```python
from build123d import *

# Parameters (mm, degrees)
SKETCH_1_R      = 2.5
EXTRUDE_1_DEPTH = 2
FILLET_1_R      = 4.5


with BuildPart() as part:
    # 草图1 → 凸台-拉伸1 (new body)
    with BuildSketch(Plane.XY):
        Polygon((-7.5, 7.5), (-7.5, -7.5), (-3, -7.5), (-3, -137.5), (-7.5, -137.5), (-7.5, -152.5), (7.5, -152.5), (7.5, -137.5), (3, -137.5), (3, -7.5), (7.5, -7.5), (7.5, 7.5), align=None)
        Circle(SKETCH_1_R, mode=Mode.SUBTRACT)
        with Locations((0, -145)):
            Circle(SKETCH_1_R, mode=Mode.SUBTRACT)
    extrude(amount=EXTRUDE_1_DEPTH)

    # 圆角1
    fillet_1_edges = [part.edges().sort_by_distance(p)[0] for p in [
        (-7.5, 7.5, 1),
        (-7.5, -7.5, 1),
        (7.5, -7.5, 1),
        (7.5, 7.5, 1),
        (7.5, -152.5, 1),
        (7.5, -137.5, 1),
        (-7.5, -152.5, 1),
        (-7.5, -137.5, 1),
    ]]
    fillet(fillet_1_edges, radius=FILLET_1_R - 0.0001)  # a hair under: the kernel refuses the full size


solid = part.part
```
Could you check a few things on this model? Use its own coordinates, in mm. A direction names the side the tool comes from. Coordinates: 2 decimals unless noted, no trailing zeros. Order: outer loops, then holes, each group sorted by start corner. A loop starts at its lowest first (then second) coordinate and runs counter-clockwise, first axis right, second up. Notation, with made-up numbers: M 38.25,9 L 78.25,9 A35 cw 78.25,46 Z; hole C -4.75,-30 d4. An arc over 180 degrees is marked long. Use a Markdown table: item, result. Add a question column.
Q1. I'm going to push a flat-ended pin straight in: pin 1 (5 mm diameter, centred on x = 4.5, y = -87.5, fed in from -Z). Where does the tip first touch, or does it pass through?
Q2. I want a section at B-B on x = 0. List the corners of the cut face in (y, z) for me, then the cut area to 3 significant figures.
Q3. I want a section at D-D on x = 6. List the corners of the cut face in (y, z) for me, then the cut area to 3 significant figures.
Q4. If I drill on L1, parallel to Y at x = 0, z = 1.35; L2, parallel to Y at x = -3.5, z = 1.6; L3, parallel to X at y = -145, z = 0.7, over which ranges is the centre line in solid material (lowest first)?
Q5. I want a section at A-A on y = -145. List the corners of the cut face in (x, z) for me.
Q6. I want a section at C-C on z = 1.2. Give the number of separate pieces and of enclosed holes in the cut face, then the cut area to 3 significant figures.
Q7. Which directions (+Z, -Z, +X, -X, +Y, -Y) give clear straight access to the entire face, cutting with the end or side of a thin tool? Please do faces 1 (the cylindrical face through (6.217, -6.147, 1.014)), 2 (the cylindrical face through (-6.217, -6.147, 1.014)), 3 (the cylindrical face through (6.147, 6.217, 1.014)).
Q8. We'd pull the mould along X, two halves only. Please class faces 4 (the flat face through (0, -71, 0)), 5 (the cylindrical face through (-6.217, 6.147, 1.014)), 6 (the cylindrical face through (-0.54, -2.44, 0.99)): pulls with the +X half, pulls with the -X half, needs draft (parallel to the pull), parting line crosses it, or undercut.
Checked values:
| question | item | result |
|---|---|---|
| 1 | pin 1 | z = 0 |
| 2 | outline | M -152.5,0 L -147.5,0 L -147.5,2 L -152.5,2 Z; M -142.5,0 L -2.5,0 L -2.5,2 L -142.5,2 Z; M 2.5,0 L 7.5,0 L 7.5,2 L 2.5,2 Z |
| 2 | area | 300 mm² |
| 3 | outline | M -151.35,0 L -138.65,0 L -138.65,2 L -151.35,2 Z; M -6.35,0 L 6.35,0 L 6.35,2 L -6.35,2 Z |
| 3 | area | 50.8 mm² |
| 4 | L1 | -152.5 to -147.5, -142.5 to -2.5, 2.5 to 7.5 |
| 4 | L2 | -152.47 to -137.53, -7.47 to 7.47 |
| 4 | L3 | -7.5 to -2.5, 2.5 to 7.5 |
| 5 | outline | M -7.5,0 L -2.5,0 L -2.5,2 L -7.5,2 Z; M 2.5,0 L 7.5,0 L 7.5,2 L 2.5,2 Z |
| 6 | separate pieces | 1 |
| 6 | enclosed holes | 2 |
| 6 | area | 1,160 mm² |
| 7 | face 1 | +Z, -Z, +X |
| 7 | face 2 | +Z, -Z, -X |
| 7 | face 3 | +Z, -Z, +X, +Y |
| 8 | face 4 | needs draft |
| 8 | face 5 | pulls with the -X half |
| 8 | face 6 | undercut |
